Build history of the part. All positions in model axes, mm. Round coordinates to 2 decimals unless told otherwise and drop trailing zeros. Loops run counter-clockwise (first coordinate to the right, second up) from the corner with the lowest first, then second, coordinate; pieces in that order, holes last. Notation, with made-up numbers: (44.5, 79.5) - (56.5, 79.5) arc R18 cw to (56.5, 108.5) - close; hole circle Ø4 at (81.25, 55.25). An arc over 180 degrees is marked (long way). Use one line per item in the form item = value. Start each with the question number.
Q1. Saw through at A-A (x = -30). Give the cut face in (y, z), then the cut area to 3 significant figures.
Q2. Pin check, flat tips, straight feed: pin 1 (2 mm diameter, centred on y = 17.5, z = 2, fed in from +X); pin 2 (1 mm diameter, centred on y = -9, z = 5.5, fed in from +X); pin 3 (1 mm diameter, centred on y = -14.5, z = 6.5, fed in from -X). Stop position of each tip, or through.
Q3. Drill centre lines: line 1 (Y direction, x = -1, z = 3.75); line 2 (X direction, y = 31, z = 0.5); line 3 (X direction, y = 26.5, z = 7). Where is each one in solid material? Low to high.
Q4. Saw through at C-C (z = 2.75). Give the cut face in (x, y).
Q5. Saw through at B-B (y = 0). Give the cut face in (x, z), then the cut area to 3 significant figures.
Q6. Saw through at D-D (x = 0). Give the cut face in (y, z).
Q7. Mould opens along X. For faces 1 (the face through (-4.88, 37.18, 3.94)), 2 (the face through (8, 1, 0)), 3 (the face through (-1.08, -4.88, 4.06)) say: released by +X, released by -X, zero draft, split by the parting line, or undercut.
```python
from build123d import *

# Parameters (mm, degrees)
SKETCH_1_R          = 37.5
EXTRUDE_1_DEPTH     = 8
SKETCH_2_R          = 4
CUT_EXTRUDE_1_DEPTH = 13
SKETCH_3_R          = 5
CUT_EXTRUDE_2_DEPTH = 13


with BuildPart() as part:
    # 草图1 → 凸台-拉伸1 (new body)
    with BuildSketch(Plane.XY):
        Circle(SKETCH_1_R)
    extrude(amount=EXTRUDE_1_DEPTH)

    # 草图2 → 切除-拉伸1 (cut)
    with BuildSketch(Plane.XY.offset(8)):
        with Locations((-30, 0)):
            Circle(SKETCH_2_R)
    extrude(amount=-CUT_EXTRUDE_1_DEPTH, mode=Mode.SUBTRACT)

    # 草图3 → 切除-拉伸2 (cut)
    with BuildSketch(Plane.XY.offset(8)):
        Circle(SKETCH_3_R)
    extrude(amount=-CUT_EXTRUDE_2_DEPTH, mode=Mode.SUBTRACT)


solid = part.part
```
Report:
q1.outline = (-22.5, 0) - (-4, 0) - (-4, 8) - (-22.5, 8) - close; (4, 0) - (22.5, 0) - (22.5, 8) - (4, 8) - close
q1.area = 296 mm²
q2.pin_1 = 33.67
q2.pin_2 = 36.52
q2.pin_3 = -34.79
q3.line_1 = -37.49 to -4.9, 4.9 to 37.49
q3.line_2 = -21.1 to 21.1
q3.line_3 = -26.53 to 26.53
q4.outline = circle Ø75 at (0, 0); hole circle Ø8 at (-30, 0); hole circle Ø10 at (0, 0)
q5.outline = (-37.5, 0) - (-34, 0) - (-34, 8) - (-37.5, 8) - close; (-26, 0) - (-5, 0) - (-5, 8) - (-26, 8) - close; (5, 0) - (37.5, 0) - (37.5, 8) - (5, 8) - close
q5.area = 456 mm²
q6.outline = (-37.5, 0) - (-5, 0) - (-5, 8) - (-37.5, 8) - close; (5, 0) - (37.5, 0) - (37.5, 8) - (5, 8) - close
q7.face_1 = split by the parting line
q7.face_2 = zero draft
q7.face_3 = undercut
